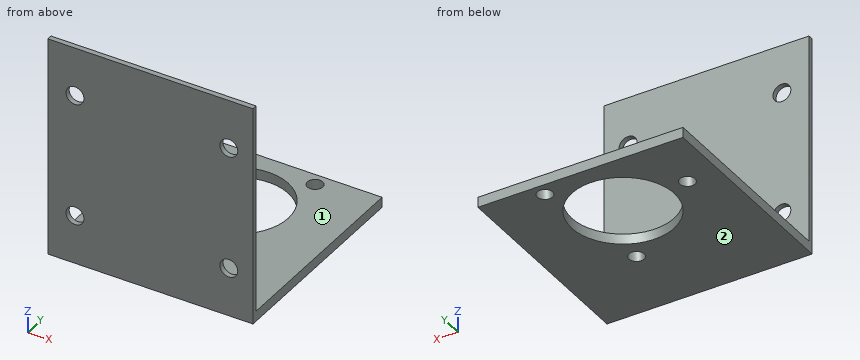
from build123d import *

# Parameters (mm, degrees)
SKETCH1_W           = 40
SKETCH1_H           = 43
SKETCH1_R           = 1.75
BOSS_EXTRUDE1_DEPTH = 1
SKETCH4_W           = 40
SKETCH4_H           = 2
BOSS_EXTRUDE2_DEPTH = 40
SKETCH5_R           = 1.5
SKETCH5_R_2         = 10
CUT_EXTRUDE1_DEPTH  = 24


with BuildPart() as part:
    # Sketch1 → Boss-Extrude1 (new body)
    with BuildSketch(Plane(origin=(0, 0, 0), x_dir=(1, 0, 0), z_dir=(0, 1, 0))):
        Rectangle(SKETCH1_W, SKETCH1_H)
        with Locations(Location((-14.715053003, 12, 0), (0, 0, 270))):
            Circle(SKETCH1_R, mode=Mode.SUBTRACT)
        with Locations(Location((15.284946997, 12, 0), (0, 0, 270))):
            Circle(SKETCH1_R, mode=Mode.SUBTRACT)
        with Locations(Location((-14.715053003, -12, 0), (0, 0, 270))):
            Circle(SKETCH1_R, mode=Mode.SUBTRACT)
        with Locations(Location((15.284946997, -12, 0), (0, 0, 270))):
            Circle(SKETCH1_R, mode=Mode.SUBTRACT)
    extrude(amount=-BOSS_EXTRUDE1_DEPTH)

    # Sketch4 → Boss-Extrude2 (add)
    with BuildSketch(Plane(origin=(0, 0, 0), x_dir=(1, 0, 0), z_dir=(0, 1, 0))):
        with Locations((0, 20.5)):
            Rectangle(SKETCH4_W, SKETCH4_H)
    extrude(amount=BOSS_EXTRUDE2_DEPTH)

    # Sketch5 → Cut-Extrude1 (cut)
    with BuildSketch(Plane.XY.offset(-19.5)):
        with Locations((8.491960292, 37.449274423)):
            Circle(SKETCH5_R)
        with Locations((-13.72832995, 28.379616129)):
            Circle(SKETCH5_R)
        with Locations((5.236369657, 13.671109447)):
            Circle(SKETCH5_R)
        with Locations((0, 26.5)):
            Circle(SKETCH5_R_2)
    extrude(amount=-CUT_EXTRUDE1_DEPTH, mode=Mode.SUBTRACT)


solid = part.part
Verification items for the finished model (mm, model axes). Face numbers are marked on the shaded views. A direction names the side the tool comes from. Give positions to 0.01 mm unless a question says otherwise; leave off trailing zeros. Loops run counter-clockwise (first coordinate to the right, second up) from the corner with the lowest first, then second, coordinate; pieces in that order, holes last.
1. Cross-section at B-B on z = -12. Record the cut outline in (x, y).
Derived:
outline: (-20, -1) - (-16.47, -1) - (-16.47, 0) - (-20, 0) - close; (-12.97, -1) - (13.53, -1) - (13.53, 0) - (-12.97, 0) - close; (17.03, -1) - (20, -1) - (20, 0) - (17.03, 0) - close
2. Cross-section at A-A on x = -7.5. Record the cut outline in (y, z), and give its area (3 significant figures).
Derived:
outline: (-1, -21.5) - (19.89, -21.5) - (19.89, -19.5) - (0, -19.5) - (0, 21.5) - (-1, 21.5) - close; (33.11, -21.5) - (40, -21.5) - (40, -19.5) - (33.11, -19.5) - close
area: 96.5 mm2
3. Cross-section at D-D on y = 27.5. Record the cut outline in (x, z).
Derived:
outline: (-20, -21.5) - (-14.94, -21.5) - (-14.94, -19.5) - (-20, -19.5) - close; (-12.51, -21.5) - (-9.95, -21.5) - (-9.95, -19.5) - (-12.51, -19.5) - close; (9.95, -21.5) - (20, -21.5) - (20, -19.5) - (9.95, -19.5) - close
4. Cross-section at C-C on y = 13. Record the cut outline in (x, z), and give its area (3 significant figures).
Derived:
outline: (-20, -21.5) - (3.89, -21.5) - (3.89, -19.5) - (-20, -19.5) - close; (6.58, -21.5) - (20, -21.5) - (20, -19.5) - (6.58, -19.5) - close
area: 74.6 mm2
5. Material ranges on probe 1 along X at (y, z) = (-0.6, -12); probe 2 along Y at (x, z) = (0, -20.35); probe 3 along Y at (x, z) = (11.5, 3.5), recorded low to high.
Derived:
probe 1: x = -20 to -16.47, -12.97 to 13.53, 17.03 to 20
probe 2: y = -1 to 16.5, 36.5 to 40
probe 3: y = -1 to 0
6. Go/stop test with flat-tipped pins: P1, Ø4, axis at x = 5, z = -4, coming from the +Y side; P2, Ø5, axis at x = 5.24, y = 13.67, coming from the +Z side. Record where each tip stops, or that it passes through.
Derived:
P1: stops at y = 0
P2: stops at z = -19.5
7. Tool access check on the marked faces 1 and 2. Record the directions out of +Z, -Z, +X, -X, +Y, -Y that give a thin tool (end or side, any length) a straight path to the whole face; none if there is none.
Derived:
face 1: +Z, +X, -X, +Y
face 2: -Z, +X, -X, +Y, -Y
